Input: part model. Units: mm. Frame: model coordinates. A direction names the side the tool comes from. Give positions to 0.01 mm unless a question says otherwise; leave off trailing zeros. Loops run counter-clockwise (first coordinate to the right, second up) from the corner with the lowest first, then second, coordinate; pieces in that order, holes last. Notation, with made-up numbers: (28.5, -15.75) - (61.5, -15.75) arc R11 ccw to (61.5, 1.25) - close; hole circle Ø2 at (79.5, -31.75). An arc over 180 degrees is marked (long way). One line per item, written item: value.
from build123d import *

# Parameters (mm, degrees)
F2_W     = 47.88
F2_H     = 47.88
F3_DEPTH = 0.31
F2_W_2   = 48.5
F2_H_2   = 48.5
F4_DEPTH = 48.5


with BuildPart() as f3:
    # F2 (on Front) → F3 (new body)
    with BuildSketch(Plane.XZ):
        with Locations((-389.1698562622, -641.3108897276)):
            Rectangle(F2_W, F2_H)
    extrude(amount=F3_DEPTH)

    # F2 (on Front) → F4 (join)
    with BuildSketch(Plane.XZ):
        with Locations((-389.1698562622, -641.3108897276)):
            Rectangle(F2_W_2, F2_H_2)
        with Locations((-389.1698562622, -641.3108897276)):
            Rectangle(F2_W, F2_H, mode=Mode.SUBTRACT)
    extrude(amount=F4_DEPTH)


solid = f3.part
Item 1: Section A-A, the plane y = -37. Output: boundary loops of the cut face in (x, z).
Verdict:
outline: (-413.42, -665.56) - (-364.92, -665.56) - (-364.92, -617.06) - (-413.42, -617.06) - close; hole (-413.11, -665.25) - (-365.23, -665.25) - (-365.23, -617.37) - (-413.11, -617.37) - close
Item 2: Pin query (flat end, axial travel): P1, Ø3, axis at x = -383.5, z = -642.5, coming from the -Y side. Return the tip coordinate at first contact, or that it passes through.
Verdict:
P1: stops at y = -0.31
Item 3: Section C-C, the plane x = -397.5. Output: boundary loops of the cut face in (y, z), and give its area (3 significant figures).
Verdict:
outline: (-48.5, -665.56) - (0, -665.56) - (0, -617.06) - (-48.5, -617.06) - (-48.5, -617.37) - (-0.31, -617.37) - (-0.31, -665.25) - (-48.5, -665.25) - close
area: 44.9 mm^2
Item 4: Material intervals for L1, parallel to X at y = -41.5, z = -633; L2, parallel to Z at x = -405.5, y = -17.5; L3, parallel to Y at x = -384.5, z = -647, sorted ascending.
Verdict:
L1: x = -413.42 to -413.11, -365.23 to -364.92
L2: z = -665.56 to -665.25, -617.37 to -617.06
L3: y = -0.31 to 0
Item 5: Section B-B, the plane z = -647. Output: boundary loops of the cut face in (x, y).
Verdict:
outline: (-413.42, -48.5) - (-413.11, -48.5) - (-413.11, -0.31) - (-365.23, -0.31) - (-365.23, -48.5) - (-364.92, -48.5) - (-364.92, 0) - (-413.42, 0) - close
Item 6: Draft query along X for faces 3 (the face through (-390, 0, -641)), 4 (the face through (-390, -0.31, -641)), 5 (the face through (-413.42, -24, -642)). Return one class per face: pulls with the +X half, pulls with the -X half, needs draft (parallel to the pull), parting line crosses it, or undercut.
Verdict:
face 3: needs draft
face 4: undercut
face 5: pulls with the -X half
Item 7: Access query for faces 1 (the face through (-390, -24, -665.251)), 2 (the face through (-390, -24, -617.061)). Directions: +Z, -Z, +X, -X, +Y, -Y. A direction counts if a zero-diameter tool reaches every point of the face in a straight line with its end or side. Return the directions, or none.
Verdict:
face 1: -Y
face 2: +Z, +X, -X, +Y, -Y
